Could you check a few things on this model? Use its own coordinates, in mm. Give positions to 0.01 mm unless a question says otherwise; leave off trailing zeros. Write each loop counter-clockwise with the first axis right and the second up, starting at its lowest first coordinate (ties: lowest second). Pieces come first, ordered by that corner, then holes. Notation, with made-up numbers: (-19.5, -9.5) - (8.5, -9.5) arc R23 cw to (8.5, 22.5) - close; hole circle Ø4 at (39, 54.25). An arc over 180 degrees is marked (long way). Write item = value, one per line.
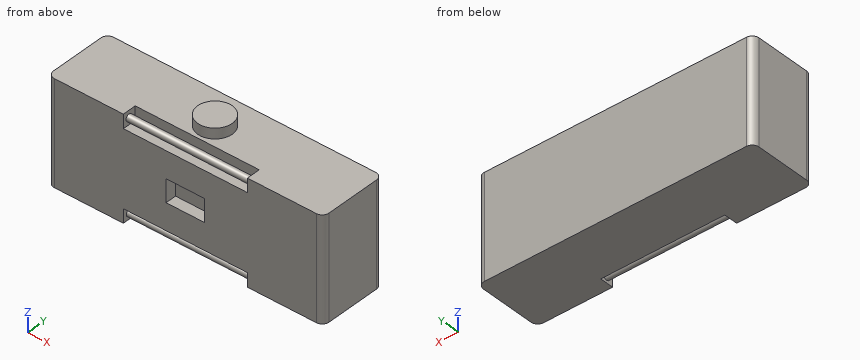
Autodesk Inventor part; units mm, degrees
ref_plane "YZ Plane" through (0, 0, 0) normal (1, 0, 0) x (0, 1, 0)
ref_plane "XZ Plane" through (0, 0, 0) normal (0, 1, 0) x (-1, 0, 0)
ref_plane "XY Plane" through (0, 0, 0) normal (0, 0, 1) x (1, 0, 0)
sketch "Sketch1" plane through (0, 0, 0) normal (0, 0, 1) x (1, 0, 0)
  line L0 (0, 1) -> (0, 9)
  line L1 (1, 10) -> (39, 10)
  line L2 (40, 9) -> (40, 1)
  line L3 (39, 0) -> (1, 0)
  arc A0 (1, 10) -> (0, 9) centre (1, 9) ccw
  arc A1 (40, 9) -> (39, 10) centre (39, 9) ccw
  arc A2 (39, 0) -> (40, 1) centre (39, 1) ccw
  arc A3 (0, 1) -> (1, 0) centre (1, 1) ccw
  point P0 (0, 0)
  point P1 (0, 10)
  point P2 (40, 10)
  point P3 (40, 0)
  dimension "d0" = 10
  dimension "d1" = 40
  dimension "d4" = 1
extrude "Extrusion1" add sketch "Sketch1" against normal blind 15
sketch "Sketch2" plane through (1, 0, 0) normal (0, -1, 0) x (1, 0, 0)
  line L0 (0, 0) -> (38, 0)
  line L1 (0, 0) -> (0, -15)
  line L2 (38, -15) -> (0, -15)
  line L3 (38, 0) -> (38, -15)
  line L4 (0, 0) -> (38, 0)
  line L5 (0, 0) -> (0, -15)
  line L6 (38, -15) -> (0, -15)
  line L7 (38, 0) -> (38, -15)
  line L8 (0, 0) -> (38, 0)
  line L9 (38, -15) -> (0, -15)
  line L10 (0, 0) -> (0, -15)
  line L11 (38, 0) -> (38, -15)
  line L12 (16.2, -5.85) -> (16.2, -9.15)
  line L13 (16.2, -9.15) -> (21.8, -9.15)
  line L14 (21.8, -9.15) -> (21.8, -5.85)
  line L15 (21.8, -5.85) -> (16.2, -5.85)
  point P0 (-1, 0)
  point P1 (16.2, -7.5)
  dimension "d8" = 3.3
  dimension "d9" = 5.6
  dimension "d10" = 16.2
  dimension "d11" = 5.85
extrude "Extrusion2" cut sketch "Sketch2" against normal blind 1.6 contours L15 L14 L13 L12
sketch "Sketch3" plane through (0, 0, 0) normal (0, 0, 1) x (1, 0, 0)
  line L0 (40, 1) -> (40, 9)
  arc A0 (40, 9) -> (39, 10) centre (39, 9) ccw
  line L1 (39, 10) -> (1, 10)
  arc A1 (1, 10) -> (0, 9) centre (1, 9) ccw
  line L2 (0, 9) -> (0, 1)
  arc A2 (0, 1) -> (1, 0) centre (1, 1) ccw
  line L3 (1, 0) -> (39, 0)
  arc A3 (39, 0) -> (40, 1) centre (39, 1) ccw
  circle A4 centre (20, 5) radius 2.5
  point P0 (0, 0)
  dimension "d14" = 5
extrude "Extrusion3" add sketch "Sketch3" along normal blind 1.5 contours A4
sketch "Sketch4" plane through (0, 0, 0) normal (0, 0, 1) x (1, 0, 0)
  line L0 (17.2, 0) -> (22.8, 0)
  line L1 (20, 0) -> (11, 0)
  line L2 (1, 0) -> (39, 0)
  line L3 (11, 0) -> (11, 2)
  line L4 (11, 2) -> (29, 2)
  line L5 (29, 2) -> (29, 0)
  line L6 (29, 0) -> (20, 0)
  point P0 (0, 0)
  point P1 (29, 0)
  dimension "d17" = 9
  dimension "d18" = 2
  dimension "d19" = 18
extrude "Extrusion4" cut sketch "Sketch4" against normal blind 2
sketch "Sketch5" plane through (0, 0, -15) normal (0, 0, -1) x (-1, 0, 0)
  line L0 (-11, 2) -> (-29, 2)
  line L1 (-11, 0) -> (-11, 2)
  line L2 (-39, 0) -> (-1, 0)
  line L3 (-29, 2) -> (-29, 0)
  point P0 (0, 0)
extrude "Extrusion5" cut sketch "Sketch5" against normal blind 2
sketch "Sketch6" plane through (11, 0, 0) normal (1, 0, 0) x (0, 0, -1)
  circle A0 centre (1.0103, 0.9523) radius 0.5
  point P0 (0, 0)
  dimension "d24" = 1
extrude "Extrusion6" add sketch "Sketch6" along normal blind 18
sketch "Sketch7" plane through (11, 0, -15) normal (1, 0, 0) x (0, 0, -1)
  circle A0 centre (-0.8887, 1) radius 0.5
  point P0 (-15, 0)
  dimension "d27" = 1
extrude "Extrusion7" add sketch "Sketch7" along normal blind 18
equation "\"BendRadius\" = Thickness"
equation "\"BendReliefWidth\" = Thickness"
equation "\"BendReliefDepth\" = 0.5 * Thickness"
equation "\"CornerReliefSize\" = 4 * Thickness"
equation "\"MinimumRemnant\" = 2 * Thickness"
equation "\"TransitionRadius\" = BendRadius"
equation "\"JacobiRadiusSize\" = BendRadius"
equation "\"GapSize\" = Thickness"
properties part number "Caja" material "Rubber, Silicone"
1. For pin 1 (0.5 mm diameter, centred on x = 21.5, y = 1, fed in from -Z); pin 2 (1.6 mm diameter, centred on x = 20, y = 0.5, fed in from +Z); pin 3 (4 mm diameter, centred on x = 11.5, y = 3.5, fed in from +Z), each with a flat end and sliding along its axis, tell me the tip position at first contact or that it passes through.
Filled sheet:
pin_1 = -14.61
pin_2 = -0.51
pin_3 = 0
2. If we section it at C-C, the plane x = 20: Please give me the cut outline in (y, z).
Filled sheet:
outline = (0, -13) - (2, -13) - (2, -15) - (10, -15) - (10, 0) - (7.5, 0) - (7.5, 1.5) - (2.5, 1.5) - (2.5, 0) - (2, 0) - (2, -2) - (0, -2) - (0, -5.85) - (1.6, -5.85) - (1.6, -9.15) - (0, -9.15) - close; circle Ø1 at (0.95, -1.01); circle Ø1 at (1, -14.11)
3. If we section it at D-D, the plane x = 9.5: Please give me the cut outline in (y, z).
Filled sheet:
outline = (0, -15) - (10, -15) - (10, 0) - (0, 0) - close
4. I need wall thicknesses on line 1 (X direction, y = 1, z = -9); line 2 (Z direction, x = 29, y = 9.5); line 3 (Y direction, x = 27, z = -1.75). Which ranges of each line are inside material? Lowest first, please.
Filled sheet:
line_1 = 0 to 17.2, 22.8 to 40
line_2 = -15 to 0
line_3 = 2 to 10
5. If we section it at A-A, the plane x = 25: Please give me the cut outline in (y, z).
Filled sheet:
outline = (0, -13) - (2, -13) - (2, -15) - (10, -15) - (10, 0) - (2, 0) - (2, -2) - (0, -2) - close; circle Ø1 at (0.95, -1.01); circle Ø1 at (1, -14.11)
6. If we section it at B-B, the plane y = 5: Please give me the cut outline in (x, z), and give its area (4 significant figures).
Filled sheet:
outline = (0, -15) - (40, -15) - (40, 0) - (22.5, 0) - (22.5, 1.5) - (17.5, 1.5) - (17.5, 0) - (0, 0) - close
area = 607.5 mm2
